```python
from build123d import *

# Parameters (mm, degrees)
F0_W        = 101.6
F0_H        = 7.62
F1_DEPTH    = 153.416
F2_W        = 7.62
F2_H        = 76.2
F3_DEPTH    = 3.302
F4_T1_DEPTH = 31.4134423739
F5_R        = 5.1053850436
F5_W        = 4.7544753179
F5_H        = 14.2634212971
F5_W_2      = 12.9049904644
F5_H_2      = 9.5089375973
F6_DEPTH    = 0.508


# Not quite as in the source:
# - a fillet or chamfer that OpenCascade refuses, or shapes differently, is made with other operations: its cross-section is extruded or revolved along the edge and cut away or added


with BuildPart() as f1:
    # F0 (on Top) → F1 (new body)
    with BuildSketch(Plane.XY):
        Rectangle(F0_W, F0_H)
    extrude(amount=F1_DEPTH)

    # F2 (on face) → F3 (join)
    with BuildSketch(Plane.XZ.offset(3.81)):
        with Locations((37.7244745995, 73.6427996308)):
            Rectangle(F2_W, F2_H)
    extrude(amount=F3_DEPTH)

    # F4: fillet of radius 5.08 on 2 edges, made by hand

    # F4_s2 → F4_t1 (cut)
    with BuildSketch(Plane.YZ.offset(22.0177534125)):
        with BuildLine():
            ThreePointArc((-3.81, 111.7427996308), (-6.2056458882, 109.8801567357), (-7.112, 106.984111156))
            Line((-7.112, 106.984111156), (-7.112, 111.7427996308))
            Line((-7.112, 111.7427996308), (-3.81, 111.7427996308))
        make_face()
        with BuildLine():
            ThreePointArc((-3.81, 35.5427996308), (-6.2056458882, 37.4054425258), (-7.112, 40.3014881055))
            Line((-7.112, 40.3014881055), (-7.112, 35.5427996308))
            Line((-7.112, 35.5427996308), (-3.81, 35.5427996308))
        make_face()
    extrude(amount=F4_T1_DEPTH, mode=Mode.SUBTRACT)

    # F5 (on face) → F6 (join)
    with BuildSketch(Plane.XZ.offset(3.81)):
        with Locations((-32.2624817491, 122.8942871094)):
            Circle(F5_R)
        with Locations((-9.5089431852, 111.3477125764)):
            Rectangle(F5_W, F5_H)
        with Locations((-31.2436651438, 77.3872062564)):
            Rectangle(F5_W_2, F5_H_2)
    extrude(amount=F6_DEPTH)


solid = f1.part
```
CAD build for the part. Positions are in the model's coordinates, mm. A direction names the side the tool comes from. Coordinates: 2 decimals unless noted, no trailing zeros. Loops run counter-clockwise (first coordinate to the right, second up) from the corner with the lowest first, then second, coordinate; pieces in that order, holes last. Notation, with made-up numbers: (-29, 45.5) - (18, 45.5) arc R19 ccw to (18, 66.5) - close; hole circle Ø2 at (17, 71). An arc over 180 degrees is marked (long way). Return JSON: item names as keys, results as strings.
1. Band-saw the part on B-B (x = -32.5). Give the cut face in (y, z).
Result:
{"outline": "(-4.32, 72.63) - (-3.81, 72.63) - (-3.81, 0) - (3.81, 0) - (3.81, 153.42) - (-3.81, 153.42) - (-3.81, 127.99) - (-4.32, 127.99) - (-4.32, 117.79) - (-3.81, 117.79) - (-3.81, 82.14) - (-4.32, 82.14) - close"}
2. Probe L1, parallel to Y at x = 36.5, z = 29; L2, parallel to X at y = -5.25, z = 93; L3, parallel to X at y = -4, z = 120.5. List the from-to ranges inside material, lowest first. Write a range as from..to.
Result:
{"L1": "y = -3.81..3.81", "L2": "x = 33.91..41.53", "L3": "x = -36.77..-27.75"}
3. 3-axis set-ups, long thin cutter, end or side, ignore diameter. For faces 1 (the flat face through (41.534, -5, 73)), 2 (the flat face through (-50.8, 0, 76)), 3 (the flat face through (-10, -4.318, 111)), 4 (the cylindrical face through (-29.52, -4.06, 127.2)): which of +Z, -Z, +X, -X, +Y, -Y reach the whole face in a straight line?
Result:
{"face 1": "+Z, -Z, +X, -Y", "face 2": "+Z, -Z, -X, +Y, -Y", "face 3": "+Z, -Z, -X, -Y", "face 4": "-Y"}
4. Band-saw the part on D-D (x = 4). Give the cut face in (y, z).
Result:
{"outline": "(-3.81, 0) - (3.81, 0) - (3.81, 153.42) - (-3.81, 153.42) - close"}
5. Band-saw the part on A-A (z = 99). Give the cut face in (x, y).
Result:
{"outline": "(-50.8, -3.81) - (33.91, -3.81) - (33.91, -7.11) - (41.53, -7.11) - (41.53, -3.81) - (50.8, -3.81) - (50.8, 3.81) - (-50.8, 3.81) - close"}
6. Band-saw the part on C-C (z = 115.5). Give the cut face in (x, y), and give its area (3 significant figures).
Result:
{"outline": "(-50.8, -3.81) - (-11.89, -3.81) - (-11.89, -4.32) - (-7.13, -4.32) - (-7.13, -3.81) - (50.8, -3.81) - (50.8, 3.81) - (-50.8, 3.81) - close", "area": "777 mm2"}
7. Drop flat-ended pins along their axis: pin 1 (12 mm diameter, centred on x = -35, z = 102.5, fed in from -Y); pin 2 (3 mm diameter, centred on x = -31.5, z = 124, fed in from -Y); pin 3 (1 mm diameter, centred on y = -6, z = 56, fed in from -X). Give the stop position or say it passes through.
Result:
{"pin 1": "stops at y = -3.81", "pin 2": "stops at y = -4.32", "pin 3": "stops at x = 33.91"}
